from build123d import *

# Parameters (mm, degrees)
SKETCH1_W             = 127
SKETCH1_H             = 152.4
BOSS_EXTRUDE1_DEPTH   = 3.175
F_8_32_TAPPED_HOLE2_D = 3.4544
SKETCH8_R             = 0.246300585
CUT_EXTRUDE1_DEPTH    = 199.40574746


with BuildPart() as part:
    # Sketch1 → Boss-Extrude1 (new body)
    with BuildSketch(Plane(origin=(0, 0, 0), x_dir=(1, 0, 0), z_dir=(0, 1, 0))):
        with Locations((63.5, 76.2)):
            Rectangle(SKETCH1_W, SKETCH1_H)
    extrude(amount=BOSS_EXTRUDE1_DEPTH)

    # #8-32 Tapped Hole2 (through all)
    with Locations(Plane(origin=(63.5, 3.175, -101.6), x_dir=(0, 0, 1), z_dir=(0, 1, 0))):
        with Locations((0, 0)):
            Hole(F_8_32_TAPPED_HOLE2_D / 2)

    # Sketch8 → Cut-Extrude1 (cut, through all)
    with BuildSketch(Plane(origin=(0, 3.175, 0), x_dir=(1, 0, 0), z_dir=(0, 1, 0))):
        with Locations(Location((52.07, 127, 0), (0, 0, 270))):
            Circle(SKETCH8_R)
        with Locations(Location((54.61, 127, 0), (0, 0, 270))):
            Circle(SKETCH8_R)
        with Locations(Location((57.15, 127, 0), (0, 0, 270))):
            Circle(SKETCH8_R)
        with Locations(Location((59.69, 127, 0), (0, 0, 270))):
            Circle(SKETCH8_R)
        with Locations(Location((62.23, 127, 0), (0, 0, 270))):
            Circle(SKETCH8_R)
        with Locations(Location((64.77, 127, 0), (0, 0, 270))):
            Circle(SKETCH8_R)
        with Locations(Location((67.31, 127, 0), (0, 0, 270))):
            Circle(SKETCH8_R)
        with Locations(Location((69.85, 127, 0), (0, 0, 270))):
            Circle(SKETCH8_R)
        with Locations(Location((72.39, 127, 0), (0, 0, 270))):
            Circle(SKETCH8_R)
        with Locations(Location((74.93, 127, 0), (0, 0, 270))):
            Circle(SKETCH8_R)
    extrude(amount=-CUT_EXTRUDE1_DEPTH, mode=Mode.SUBTRACT)


solid = part.part
Build history of the part. All positions in model axes, mm. Round coordinates to 2 decimals unless told otherwise and drop trailing zeros. Write each loop counter-clockwise with the first axis right and the second up, starting at its lowest first coordinate (ties: lowest second). Pieces come first, ordered by that corner, then holes. Notation, with made-up numbers: M 15,66 L 54,66 A17 ccw 54,83 Z; hole C 33.5,8 d5. An arc over 180 degrees is marked long. Use CSV: the item, a comma, the result in double quotes.
1. Saw through at A-A (z = -101.6). Give the cut face in (x, y) (3 decimals).
Reply:
outline,"M 0,0 L 61.773,0 L 61.773,3.175 L 0,3.175 Z; M 65.227,0 L 127,0 L 127,3.175 L 65.227,3.175 Z"
2. Two-plate mould, pull along Z, no slides. Class faces 1 (the face through (127, 2, -75)), 2 (the face through (63, 2, -152.4)), 3 (the face through (63.576, 1.565, -99.874)): +Z half, -Z half, draft (parallel to the pull), parting line (faces both ways), or undercut.
Reply:
face 1,"draft"
face 2,"-Z half"
face 3,"undercut"
3. Wall check: probe 1 along Z at (x, y) = (59.69, 2.3); probe 2 along Z at (x, y) = (64.77, 1.05). Give the ranges that are in metal, low to high. Write a range as from..to.
Reply:
probe 1,"z = -152.4..-127.25, -126.75..0"
probe 2,"z = -152.4..-127.25, -126.75..-102.77, -100.43..0"
